Input: part model. Units: mm. Frame: model coordinates. Give positions to 0.01 mm unless a question says otherwise; leave off trailing zeros. Loops run counter-clockwise (first coordinate to the right, second up) from the corner with the lowest first, then second, coordinate; pieces in that order, holes last. Notation, with made-up numbers: (-11, -27) -> (30, -27) arc R9 ccw to (30, -10) -> close; hole circle Ø10 at (74.25, 10). An arc over 180 degrees is marked (long way). Answer as a JSON object with one key per item and string values. Group by question number.
Autodesk Fusion 360 part; units mm, degrees
sketch "草图8" plane through (0, 0, 0) normal (0, 0, 1) x (1, 0, 0)
  line L0 (-8.5, 10) -> (8.5, 10)
  line L1 (8.5, 10) -> (8.5, -10)
  line L2 (8.5, -10) -> (-8.5, -10)
  line L3 (-8.5, -10) -> (-8.5, 10)
  line L4 (0, 1.75) -> (0, 22.5)
  line L5 (1.75, 0) -> (22.5, 0)
  dimension "d5" = 17
  dimension "d6" = 20
extrude "拉伸5" add sketch "草图8" along normal blind 200
fillet "圆角2" radius 10 2 edges at (0, -10, 200) (0, 10, 200)
sketch "草图10" plane through (8.5, 0, 0) normal (1, 0, 0) x (0, 1, 0)
  arc A0 (10, 190) -> (-10, 190) centre (0, 190) ccw
  line L0 (-10, 190) -> (-10, 0)
  line L1 (-10, 0) -> (10, 0)
  line L2 (10, 0) -> (10, 190)
  circle A1 centre (0, 180) radius 3.5
  dimension "d14" = 7
  dimension "d15" = 180
extrude "拉伸6" cut sketch "草图10" against normal blind 175 contours A1
Q1. Ray query, probe 1 along Y at (x, z) = (4.5, 180); probe 2 along Z at (x, y) = (4.5, 0); probe 3 along Z at (x, y) = (1.75, 0.75). Return the intervals inside material, ascending.
Q2. Section B-B on y = -8.25. Return the cut outline in (x, z).
Q3. Section A-A on z = 180. Return the cut outline in (x, y), then the cut area to 3 significant figures.
Q4. Pull-direction query (Y, two-part tool) for faces 1 (the face through (0, -10, 94)), 2 (the face through (0.119, -0.759, 176.583)), 3 (the face through (0, 10, 99)); classes: +Y half, -Y half, draft (parallel to the pull), parting line (faces both ways), or undercut.
Q5. Pin query (flat end, axial travel): pin 1 Ø6 at (x, y) = (4.5, -6.5) entering from +Z. Return the tip coordinate at first contact, or that it passes through.
Numbers:
{
 "1": {"probe 1": "y = -10 to -3.5, 3.5 to 10", "probe 2": "z = 0 to 176.5, 183.5 to 200", "probe 3": "z = 0 to 176.58, 183.42 to 200"},
 "2": {"outline": "(-8.5, 0) -> (8.5, 0) -> (8.5, 195.65) -> (-8.5, 195.65) -> close"},
 "3": {"outline": "(-8.5, -10) -> (8.5, -10) -> (8.5, -3.5) -> (-8.5, -3.5) -> close; (-8.5, 3.5) -> (8.5, 3.5) -> (8.5, 10) -> (-8.5, 10) -> close", "area": "221 mm²"},
 "4": {"face 1": "-Y half", "face 2": "undercut", "face 3": "+Y half"},
 "5": {"pin 1": "stops at z = 199.37"}
}
